Build history of the part. All positions in model axes, mm. A direction names the side the tool comes from. Coordinates: 2 decimals unless noted, no trailing zeros. Order: outer loops, then holes, each group sorted by start corner. A loop starts at its lowest first (then second) coordinate and runs counter-clockwise, first axis right, second up. Notation, with made-up numbers: M -22,3.25 L 22,3.25 A8 cw 22,14.25 Z; hole C 44.25,-5.75 d5. An arc over 180 degrees is marked long. Write item = value, one per line. Start each with the question number.
Q1. Band-saw the part on A-A on x = -20. Write the cut outline in (y, z), plus the area to 3 significant figures.
Q2. Pull direction Z, two halves, no side cores. Call faces 3 (the face through (-25, -13, -13.477)), 4 (the face through (-19, 0, 4)), 5 (the face through (-37.16, -10.06, 4.98)): released by +Z, released by -Z, zero draft, split by the parting line, or undercut.
Q3. Band-saw the part on B-B on z = 14. Write the cut outline in (x, y), plus the area to 3 significant figures.
Q4. 3-axis set-ups, long thin cutter, end or side, ignore diameter. For faces 1 (the face through (3.651, -6, 8)), 2 (the face through (-14.28, -19.14, -4.32)): which of +Z, -Z, +X, -X, +Y, -Y reach the whole face in a straight line?
Q5. Drill centre lines: probe 1 along Y at (x, z) = (-15, 23); probe 2 along X at (y, z) = (-4.5, 21); probe 3 along X at (y, z) = (-6.75, 3.5). Where is each one in solid material? Low to high.
Q6. Band-saw the part on C-C on y = -16. Write the cut outline in (x, z), plus the area to 3 significant figures.
Q7. Band-saw the part on D-D on x = -4.5. Write the cut outline in (y, z), plus the area to 3 significant figures.
```python
from build123d import *

# Parameters (mm, degrees)
F0_W     = 57.15
F0_H     = 44.45
F1_DEPTH = 25.4
F2_R     = 11.414104
F3_DEPTH = 25.4
F5_DEPTH = 12.7


with BuildPart() as f1:
    # F0 (on Front) → F1 (new body)
    with BuildSketch(Plane.XZ):
        with Locations((-24.923741, 8.748023)):
            Rectangle(F0_W, F0_H)
    extrude(amount=F1_DEPTH)

    # F2 (on face) → F3 (cut)
    with BuildSketch(Plane.XZ.offset(25.4)):
        with Locations((-28.098741, 11.923023)):
            Circle(F2_R)
    extrude(amount=-F3_DEPTH, mode=Mode.SUBTRACT)

    # F4 (on face) → F5 (cut)
    with BuildSketch(Plane.XZ.offset(25.4)):
        Polygon((3.651259, 30.973023), (-34.448741, 30.973023), (-9.048741, -13.476977), (3.651259, -13.476977), align=None)
    extrude(amount=-F5_DEPTH, mode=Mode.SUBTRACT)


solid = f1.part
```
Recorded:
q1.outline = M -25.4,-13.48 L 0,-13.48 L 0,3.88 L -25.4,3.88 Z; M -12.7,19.97 L 0,19.97 L 0,30.97 L -12.7,30.97 Z
q1.area = 581 mm2
q2.face_3 = released by -Z
q2.face_4 = zero draft
q2.face_5 = undercut
q3.outline = M -53.5,-25.4 L -39.32,-25.4 L -39.32,0 L -53.5,0 Z; M -16.88,-12.7 L 3.65,-12.7 L 3.65,0 L -16.88,0 Z
q3.area = 621 mm2
q4.face_1 = +Z, -Z, +X, +Y, -Y
q4.face_2 = +Z, +X, -Y
q5.probe_1 = -12.7 to 0
q5.probe_2 = -53.5 to -35.02, -21.18 to 3.65
q5.probe_3 = -53.5 to -35.8, -20.4 to 3.65
q6.outline = M -53.5,-13.48 L -9.05,-13.48 L -19.36,4.58 A11.41 cw long -29.99,23.18 L -34.45,30.97 L -53.5,30.97 Z
q6.area = 1,120 mm2
q7.outline = M -12.7,-13.48 L 0,-13.48 L 0,30.97 L -12.7,30.97 Z
q7.area = 565 mm2
